```python
from build123d import *

# Parameters (mm, degrees)
SKETCH1_R           = 6.469950333
BOSS_EXTRUDE1_DEPTH = 10


with BuildPart() as part:
    # Sketch1 → Boss-Extrude1 (new body)
    with BuildSketch(Plane.XY):
        Polygon((0, 0), (-34.094374575, 42.711992732), (190.731046947, 222.176392423), (224.825421522, 179.464399691), align=None)
        with Locations((35.743173778, 65.760421737)):
            Circle(SKETCH1_R, mode=Mode.SUBTRACT)
        with Locations((114.698226452, 125.411384111)):
            Circle(SKETCH1_R, mode=Mode.SUBTRACT)
        with Locations((183.769608582, 180.906879578)):
            Circle(SKETCH1_R, mode=Mode.SUBTRACT)
    extrude(amount=BOSS_EXTRUDE1_DEPTH)


solid = part.part
```
Could you check a few things on this model? Use its own coordinates, in mm. Coordinates: 2 decimals unless noted, no trailing zeros. Write each loop counter-clockwise with the first axis right and the second up, starting at its lowest first coordinate (ties: lowest second). Pieces come first, ordered by that corner, then holes. Notation, with made-up numbers: M -39.5,8 L -24.5,8 A30 ccw -24.5,30 Z; hole C 45,27 d8. An arc over 180 degrees is marked long. Answer as CSV lines item,"result". Start each with the question number.
1) Please list where these lines run through material, in increasing order: line 1 (Y direction, x = 32, z = 3.75); line 2 (X direction, y = 176, z = 9.25); line 3 (Y direction, x = 112.5, z = 4.75). Write a range as from..to.
2) I want a section at C-C, the plane x = 111. Please give me the cut outline in (y, z).
3) We'd pull the mould along X, two halves only. Please class faces 1 (the flat face through (114, 91, 5)), 2 (the flat face through (-16.81, 21.06, 4.93)), 3 (the cylindrical face through (34.341, 59.444, 4.93)): +X half, -X half, draft (parallel to the pull), parting line (faces both ways), or undercut.
4) I want a section at B-B, the plane z = 8. Please give me the cut outline in (x, y), and give its area (3 significant figures).
5) I want a section at A-A, the plane x = 34.5. Please give me the cut outline in (y, z).
6) For P1, Ø1, axis at x = 136.5, y = 150, coming from the -Z side; P2, Ø5, axis at y = 123.5, z = 2, coming from the -X side; P3, Ø4, axis at x = 141, z = 6, coming from the -Y side; P4, Ø1.5, axis at x = 63, z = 1, coming from the +Y side, each with a flat end and sliding along its axis, tell me the tip position at first contact or that it passes through.
7) I want a section at D-D, the plane y = 26.5. Please give me the cut outline in (x, z).
Data:
1,line 1,"y = 25.54..60.48, 71.04..95.47"
1,line 2,"x = 132.88..179.55, 187.99..220.49"
1,line 3,"y = 89.8..119.33, 131.5..159.73"
2,outline,"M 88.6,0 L 120.1,0 L 120.1,10 L 88.6,10 Z; M 130.72,0 L 158.53,0 L 158.53,10 L 130.72,10 Z"
3,face 1,"+X half"
3,face 2,"-X half"
3,face 3,"undercut"
4,outline,"M -34.09,42.71 L 0,0 L 224.83,179.46 L 190.73,222.18 Z; hole C 35.74,65.76 d12.94; hole C 114.7,125.41 d12.94; hole C 183.77,180.91 d12.94"
4,area,"15,300 mm^2"
5,outline,"M 27.54,0 L 59.41,0 L 59.41,10 L 27.54,10 Z; M 72.11,0 L 97.47,0 L 97.47,10 L 72.11,10 Z"
6,P1,"stops at z = 0"
6,P2,"stops at x = 63.98"
6,P3,"stops at y = 110.96"
6,P4,"stops at y = 120.82"
7,outline,"M -21.15,0 L 33.2,0 L 33.2,10 L -21.15,10 Z"
